from build123d import *

# Parameters (mm, degrees)
BOSS_EXTRUDE1_DEPTH                             = 37.5
FILLET1_R                                       = 5.969
SKETCH2_R                                       = 21
CUT_EXTRUDE1_DEPTH                              = 21
CIRPATTERN1_COUNT                               = 4
SKETCH5_R                                       = 15
CUT_EXTRUDE2_DEPTH                              = 21
CSK_FOR_M8_FLAT_HEAD_MACHINE_SCREW1_D           = 8.4
CSK_FOR_M8_FLAT_HEAD_MACHINE_SCREW1_DEPTH       = 12.7
CSK_FOR_M8_FLAT_HEAD_MACHINE_SCREW1_CSINK_D     = 17.3
CSK_FOR_M8_FLAT_HEAD_MACHINE_SCREW1_CSINK_ANGLE = 90
CSK_FOR_M8_FLAT_HEAD_MACHINE_SCREW1_TIP         = 2.5236146
M6_CLEARANCE_HOLE1_D                            = 6.4
M6_CLEARANCE_HOLE1_DEPTH                        = 12.7
M6_CLEARANCE_HOLE1_TIP                          = 1.922753981
SKETCH13_R                                      = 3
SKETCH13_R_2                                    = 4
CUT_EXTRUDE3_DEPTH                              = 11.938


with BuildPart() as part:
    # Sketch1 → Boss-Extrude1 (new body, symmetric)
    with BuildSketch(Plane.XY):
        Polygon((-140.462, 101.6), (-152.4, 101.6), (-152.4, 0), (152.4, 0), (152.4, 101.6), (140.462, 101.6), (140.462, 7.366), (-140.462, 7.366), align=None)
    extrude(amount=BOSS_EXTRUDE1_DEPTH, both=True)

    # Fillet1
    fillet1_edges = [part.edges().sort_by_distance(p)[0] for p in [
        (-140.462, 7.366, 0),
        (140.462, 7.366, 0),
        (140.462, 101.6, 0),
        (-140.462, 101.6, 0),
    ]]
    fillet(fillet1_edges, radius=FILLET1_R)

    # Sketch2 → Cut-Extrude1 (cut)
    with BuildSketch(Plane(origin=(152.4, 0, 0), x_dir=(0, 0, -1), z_dir=(1, 0, 0))):
        with Locations((0, 70)):
            Circle(SKETCH2_R)
    extrude(amount=-CUT_EXTRUDE1_DEPTH, mode=Mode.SUBTRACT)

    # Sketch4 → CSK for M5 Flat Head Machine Screw1 (revolve, cut)
    with BuildSketch(Plane(origin=(140.462, 88.384776311, 18.384776311), x_dir=(0, 0, 1), z_dir=(0, 1, 0))):
        Polygon((0, 0), (0, 20.59228064), (2.65, 19), (2.65, 2.55), (5.2, 0), align=None)
    csk_for_m5_flat_head_machine_screw1 = revolve(axis=Axis((134.112, 88.384776311, 18.384776311), (1, 0, 0)), mode=Mode.SUBTRACT)

    # CirPattern1: CSK for M5 Flat Head Machine Screw1 ×4 about axis
    cirpattern1_axis = Axis((0, 70, 0), (1, 0, 0))
    for i in range(1, CIRPATTERN1_COUNT):
        add(csk_for_m5_flat_head_machine_screw1.rotate(cirpattern1_axis, i * 360 / CIRPATTERN1_COUNT), mode=Mode.SUBTRACT)

    # Sketch5 → Cut-Extrude2 (cut)
    with BuildSketch(Plane(origin=(-140.462, 0, 0), x_dir=(0, 0, -1), z_dir=(1, 0, 0))):
        with Locations((0, 70)):
            Circle(SKETCH5_R)
    extrude(amount=-CUT_EXTRUDE2_DEPTH, mode=Mode.SUBTRACT)

    # CSK for M8 Flat Head Machine Screw1
    with Locations(Plane(origin=(-19.12664, 0, 26.5), x_dir=(0, 0, -1), z_dir=(0, -1, 0))):
        with Locations((0, 0), (0, 53), (53, 53), (53, 0)):
            CounterSinkHole(CSK_FOR_M8_FLAT_HEAD_MACHINE_SCREW1_D / 2, CSK_FOR_M8_FLAT_HEAD_MACHINE_SCREW1_CSINK_D / 2, depth=CSK_FOR_M8_FLAT_HEAD_MACHINE_SCREW1_DEPTH, counter_sink_angle=CSK_FOR_M8_FLAT_HEAD_MACHINE_SCREW1_CSINK_ANGLE)
            with Locations((0, 0, -(CSK_FOR_M8_FLAT_HEAD_MACHINE_SCREW1_DEPTH + CSK_FOR_M8_FLAT_HEAD_MACHINE_SCREW1_TIP / 2))):  # 118° drill point
                Cone(0, CSK_FOR_M8_FLAT_HEAD_MACHINE_SCREW1_D / 2, CSK_FOR_M8_FLAT_HEAD_MACHINE_SCREW1_TIP, mode=Mode.SUBTRACT)

    # M6 Clearance Hole1
    with Locations(Plane(origin=(-120, 0, 27.5), x_dir=(0, 0, -1), z_dir=(0, -1, 0))):
        with Locations((0, 0), (0, 240), (55, 240), (55, 0)):
            Hole(M6_CLEARANCE_HOLE1_D / 2, depth=M6_CLEARANCE_HOLE1_DEPTH)
            with Locations((0, 0, -(M6_CLEARANCE_HOLE1_DEPTH + M6_CLEARANCE_HOLE1_TIP / 2))):  # 118° drill point
                Cone(0, M6_CLEARANCE_HOLE1_D / 2, M6_CLEARANCE_HOLE1_TIP, mode=Mode.SUBTRACT)

    # Sketch13 → Cut-Extrude3 (cut)
    with BuildSketch(Plane.ZY.offset(152.4)):
        with Locations((-18.384776311, 88.384776311)):
            Circle(SKETCH13_R)
        with Locations((18.384776311, 51.615223689)):
            Circle(SKETCH13_R)
        with Locations((-14.849242405, 55.150757595)):
            Circle(SKETCH13_R_2)
        with Locations((14.849242405, 84.849242405)):
            Circle(SKETCH13_R_2)
    extrude(amount=-CUT_EXTRUDE3_DEPTH, mode=Mode.SUBTRACT)


solid = part.part
Can you work these out from the model? Positions are in its coordinate system, mm. A direction names the side the tool comes from. Round coordinates to 2 decimals unless told otherwise and drop trailing zeros. Order: outer loops, then holes, each group sorted by start corner. A loop starts at its lowest first (then second) coordinate and runs counter-clockwise, first axis right, second up. Notation, with made-up numbers: M -18.5,30 L 36.5,30 A13 cw 36.5,34 Z; hole C 40,88.5 d8. An arc over 180 degrees is marked long. Use a Markdown table: item, result.
1) Imagine slicing it at B-B (z = 0). List the corners of the cut face in (x, y) for me (3 decimals), then the cut area to 3 significant figures.
Geometry says:
| item | result |
|---|---|
| outline | M -152.4,0 L 152.4,0 L 152.4,49 L 140.462,49 L 140.462,13.335 A5.969 cw 134.493,7.366 L -134.493,7.366 A5.969 cw -140.462,13.335 L -140.462,55 L -152.4,55 Z; M -152.4,85 L -140.462,85 L -140.462,95.631 A5.969 ccw -146.431,101.6 L -152.4,101.6 Z; M 140.462,91 L 152.4,91 L 152.4,101.6 L 146.431,101.6 A5.969 ccw 140.462,95.631 Z |
| area | 3,640 mm² |
2) If I drill on line 1 along X through (y, z) = (5, -27); line 2 along X through (y, z) = (59.5, 33.5); line 3 along Y through (x, z) = (146.5, 0), over which ranges is the centre line in solid material (lowest first)?
Geometry says:
| item | result |
|---|---|
| line 1 | x = -152.4 to -123.16, -116.84 to -23.3, -14.96 to 29.7, 38.04 to 116.84, 123.16 to 152.4 |
| line 2 | x = -152.4 to -140.46, 140.46 to 152.4 |
| line 3 | y = 0 to 49, 91 to 101.6 |
3) If we mould it in two halves opening along X, with no side actions, what happens to faces 1 (the face through (147.64, 90.833, -19.4)), 2 (the face through (-118, 4, 25)), 3 (the face through (152.4, 39, 1)), 4 (the face through (29.773, 5.928, -27.41))? For each: +X half, -X half, draft (parallel to the pull), parting line (faces both ways), or undercut.
Geometry says:
| item | result |
|---|---|
| face 1 | draft |
| face 2 | undercut |
| face 3 | +X half |
| face 4 | undercut |
4) Imagine slicing it at C-C (y = 70). List the corners of the cut face in (x, z) for me.
Geometry says:
| item | result |
|---|---|
| outline | M -152.4,-37.5 L -140.46,-37.5 L -140.46,-15 L -152.4,-15 Z; M -152.4,15 L -140.46,15 L -140.46,37.5 L -152.4,37.5 Z; M 140.46,-37.5 L 152.4,-37.5 L 152.4,-21 L 140.46,-21 Z; M 140.46,21 L 152.4,21 L 152.4,37.5 L 140.46,37.5 Z |
5) Imagine slicing it at D-D (y = 23). List the corners of the cut face in (x, z) for me, then the cut area to 3 significant figures.
Geometry says:
| item | result |
|---|---|
| outline | M -152.4,-37.5 L -140.46,-37.5 L -140.46,37.5 L -152.4,37.5 Z; M 140.46,-37.5 L 152.4,-37.5 L 152.4,37.5 L 140.46,37.5 Z |
| area | 1,790 mm² |
6) Imagine slicing it at A-A (x = -120). List the corners of the cut face in (y, z) for me, then the cut area to 3 significant figures.
Geometry says:
| item | result |
|---|---|
| outline | M 0,-37.5 L 7.37,-37.5 L 7.37,-30.7 L 0,-30.7 Z; M 0,-24.3 L 7.37,-24.3 L 7.37,24.3 L 0,24.3 Z; M 0,30.7 L 7.37,30.7 L 7.37,37.5 L 0,37.5 Z |
| area | 458 mm² |
7) On a 3-axis mill with a long thin cutter (end or side, diameter ignored), from which of +Z, -Z, +X, -X, +Y, -Y can I reach the whole of each face in a straight line? I mean faces 5 (the face through (142.852, 50.539, -20.98)), 6 (the face through (147.64, 52.411, -20.912)), 7 (the face through (-17.8, 4.234, 30.712)), 8 (the face through (-146.515, 52.717, -18.024)). Say none if no direction works.
Geometry says:
| item | result |
|---|---|
| face 5 | none |
| face 6 | +X |
| face 7 | -Y |
| face 8 | -X |
8) I'm going to push flat-ended pins straight in: P1, Ø10, axis at x = -4.5, z = -23.5, coming from the +Y side; P2, Ø5, axis at y = 51.62, z = 18.38, coming from the -X side; P3, Ø13.5, axis at x = -19.13, z = -26.5, coming from the -Y side. Where does each tip first touch, or does it pass through?
Geometry says:
| item | result |
|---|---|
| P1 | stops at y = 7.37 |
| P2 | passes through |
| P3 | stops at y = 1.9 |
